Part model, mm, in its own coordinate system. Face numbers are marked on the shaded views. A direction names the side the tool comes from. Give positions to 0.01 mm unless a question says otherwise; leave off trailing zeros. Order: outer loops, then holes, each group sorted by start corner. A loop starts at its lowest first (then second) coordinate and runs counter-clockwise, first axis right, second up. Notation, with made-up numbers: (31.25, -25.5) - (57.25, -25.5) arc R15 ccw to (57.25, -18.5) - close; hole circle Ø5 at (-8, 24.5). An arc over 180 degrees is marked (long way). Use a Markdown table: item, result. Add a question column.
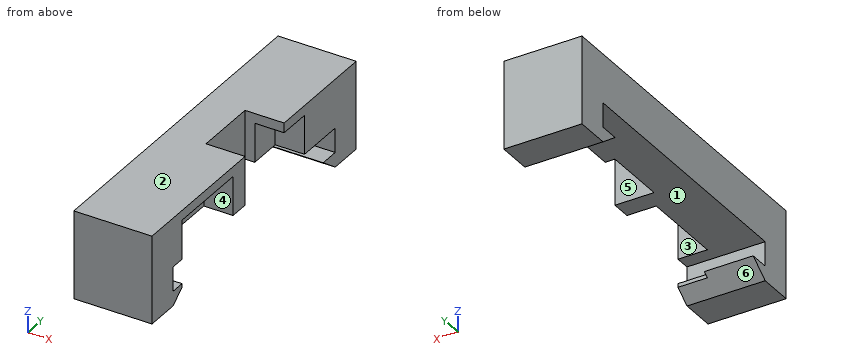
from build123d import *

# Parameters (mm, degrees)
SKETCH1_W           = 4
SKETCH1_H           = 17
BOSS_EXTRUDE1_DEPTH = 6
SKETCH2_W           = 2
SKETCH2_H           = 3.25
SKETCH2_W_2         = 1.5
SKETCH2_H_2         = 1.25
CUT_EXTRUDE1_DEPTH  = 19.466185313
CUT_EXTRUDE2_DEPTH  = 19.466185313
SKETCH4_W           = 2
SKETCH4_H           = 1.25
BOSS_EXTRUDE2_DEPTH = 2
BOSS_EXTRUDE3_DEPTH = 2
SKETCH6_W           = 1.5
SKETCH6_H           = 1.7
SKETCH6_H_2         = 4
CUT_EXTRUDE3_DEPTH  = 2
SKETCH7_W           = 4
SKETCH7_H           = 17
CUT_EXTRUDE4_DEPTH  = 10
SKETCH8_W           = 1.5
SKETCH8_H           = 1
BOSS_EXTRUDE4_DEPTH = 2


with BuildPart() as part:
    # Sketch1 → Boss-Extrude1 (new body)
    with BuildSketch(Plane.XY):
        with Locations((2, 8.5)):
            Rectangle(SKETCH1_W, SKETCH1_H)
    extrude(amount=BOSS_EXTRUDE1_DEPTH)

    # Sketch2 → Cut-Extrude1 (cut, through all)
    with BuildSketch(Plane.XY.offset(6)):
        with Locations((3, 9.375)):
            Rectangle(SKETCH2_W, SKETCH2_H)
        with Locations((3.25, 3.125)):
            Rectangle(SKETCH2_W_2, SKETCH2_H_2)
    extrude(amount=-CUT_EXTRUDE1_DEPTH, mode=Mode.SUBTRACT)

    # Sketch3 → Cut-Extrude2 (cut, through all)
    with BuildSketch(Plane.ZY):
        Polygon((0, 15.25), (0.75, 14.25), (0.75, 15.25), (2, 15.25), (2, 1.75), (0.75, 1.75), (0.75, 2.75), (0, 1.75), align=None)
    extrude(amount=-CUT_EXTRUDE2_DEPTH, mode=Mode.SUBTRACT)

    # Sketch4 → Boss-Extrude2 (add)
    with BuildSketch(Plane(origin=(4, 0, 0), x_dir=(0, 0, -1), z_dir=(1, 0, 0))):
        with Locations((-5, 3.125)):
            Rectangle(SKETCH4_W, SKETCH4_H)
    extrude(amount=-BOSS_EXTRUDE2_DEPTH)

    # Sketch5 → Boss-Extrude3 (add)
    with BuildSketch(Plane.XY.offset(6)):
        Polygon((0, 14.5), (2, 14.5), (2, 12.2), (4, 12.2), (4, 11), (2, 11), (2, 7.75), (4, 7.75), (4, 6.55), (2, 6.55), (2, 2.5), (0, 2.5), align=None)
    extrude(amount=BOSS_EXTRUDE3_DEPTH)

    # Sketch6 → Cut-Extrude3 (cut)
    with BuildSketch(Plane(origin=(0, 0, 2), x_dir=(-1, 0, 0), z_dir=(0, 0, -1))):
        with Locations((-3.25, 11.85)):
            Rectangle(SKETCH6_W, SKETCH6_H)
        with Locations((-3.25, 5.75)):
            Rectangle(SKETCH6_W, SKETCH6_H_2)
    extrude(amount=-CUT_EXTRUDE3_DEPTH, mode=Mode.SUBTRACT)

    # Sketch7 → Cut-Extrude4 (cut)
    with BuildSketch(Plane(origin=(4, 0, 0), x_dir=(0, 0, -1), z_dir=(1, 0, 0))):
        with Locations((-6.5, 8.5)):
            Rectangle(SKETCH7_W, SKETCH7_H)
    extrude(amount=-CUT_EXTRUDE4_DEPTH, mode=Mode.SUBTRACT)

    # Sketch8 → Boss-Extrude4 (add)
    with BuildSketch(Plane(origin=(0, 0, 4), x_dir=(-1, 0, 0), z_dir=(0, 0, -1))):
        with Locations((-3.25, 7.25)):
            Rectangle(SKETCH8_W, SKETCH8_H)
    extrude(amount=BOSS_EXTRUDE4_DEPTH)


solid = part.part
1. Cut at A-A (x = 2.7). Write the cut outline in (y, z).
2. Cut at C-C (y = 4.25). Write the cut outline in (x, z), plus the area to 3 significant figures.
3. Cut at D-D (x = 0.8). Write the cut outline in (y, z).
4. Drill centre lines: probe 1 along Y at (x, z) = (2.75, 2.9); probe 2 along Y at (x, z) = (2.4, 1.9); probe 3 along Y at (x, z) = (2.15, 3.95). Where is each one in solid material? Low to high. Write a range as [from, to].
5. Tool access for the marked faces 4, 5 and 6: list every direction of +Z, -Z, +X, -X, +Y, -Y with a clear straight run to the whole face (end or side of a thin tool).
6. Cut at B-B (z = 1.5). Write the cut outline in (x, y).
7. Mould opens along Z. For the marked faces 1, 2 and 3 say: released by +Z, released by -Z, zero draft, split by the parting line, or undercut.
8. Pin check, flat tips, straight feed: P1, Ø2, axis at y = 9.5, z = 3.5, coming from the +X side; P2, Ø1.6, axis at x = 3, z = 3, coming from the -Y side; P3, Ø1.2, axis at x = 2, y = 7.5, coming from the -Z side. Stop position of each tip, or through.
Responses:
| question | item | result |
|---|---|---|
| 1 | outline | (0, 0) - (1.75, 0) - (2.5, 0.56) - (2.5, 0.75) - (1.75, 0.75) - (1.75, 2) - (2.5, 2) - (2.5, 4) - (6.75, 4) - (6.75, 2) - (7.75, 2) - (7.75, 4.5) - (0, 4.5) - close; (11, 4) - (12.7, 4) - (12.7, 2) - (15.25, 2) - (15.25, 0.75) - (14.25, 0.75) - (15.25, 0) - (17, 0) - (17, 4.5) - (11, 4.5) - close |
| 2 | outline | (0, 2) - (2.5, 2) - (2.5, 4) - (4, 4) - (4, 4.5) - (0, 4.5) - close |
| 2 | area | 7.00 mm² |
| 3 | outline | (0, 0) - (1.75, 0) - (2.75, 0.75) - (1.75, 0.75) - (1.75, 2) - (15.25, 2) - (15.25, 0.75) - (14.25, 0.75) - (15.25, 0) - (17, 0) - (17, 4.5) - (0, 4.5) - close |
| 4 | probe 1 | y = [0, 2.5], [6.75, 7.75], [12.7, 17] |
| 4 | probe 2 | y = [0, 1.75], [15.25, 17] |
| 4 | probe 3 | y = [0, 7.75], [11, 17] |
| 5 | face 4 | -Z, +X |
| 5 | face 5 | +Z, -Z, +X |
| 5 | face 6 | -Z, +X, -X |
| 6 | outline | (0, 0) - (4, 0) - (4, 1.75) - (0, 1.75) - close; (0, 15.25) - (4, 15.25) - (4, 17) - (0, 17) - close |
| 7 | face 1 | undercut |
| 7 | face 2 | released by +Z |
| 7 | face 3 | zero draft |
| 8 | P1 | stops at x = 2 |
| 8 | P2 | stops at y = 0 |
| 8 | P3 | stops at z = 2 |
